Model file for the job. Use its own axes, mm. A direction names the side the tool comes from. Round coordinates to 2 decimals unless told otherwise and drop trailing zeros. Loops run counter-clockwise (first coordinate to the right, second up) from the corner with the lowest first, then second, coordinate; pieces in that order, holes last. Notation, with made-up numbers: (54, 22.5) - (107, 22.5) arc R17 cw to (107, 27.5) - close; hole circle Ø11 at (32.25, -37). An arc over 180 degrees is marked (long way). Answer as a JSON object with one key per item and string values.
from build123d import *

# Parameters (mm, degrees)
F3_DEPTH  = 533.4
F5_DEPTH  = 330.2
F6_W      = 895.4597115517
F6_H      = 69.037437439
F7_DEPTH  = 254
F9_DEPTH  = 152.4
F11_W     = 951.6055583954
F11_H     = 58.4162473679
F12_DEPTH = 254
F13_R     = 205.1226496696
F14_DEPTH = 203.2
F16_DEPTH = 203.2
F17_W     = 673.4294295311
F17_H     = 270.8390951157
F18_DEPTH = 254
F20_DEPTH = 228.6
F22_DEPTH = 50.8
F23_W     = 39.8923233151
F23_H     = 31.9777131081
F24_DEPTH = 50.8
F25_R     = 128.4316644383
F26_DEPTH = 25.4


with BuildPart() as f3:
    # F2 (on face) → F3 (new body, symmetric)
    with BuildSketch(Plane.YZ):
        Polygon((580.4695487022, 438.6440515518), (954.6338915825, 438.6440515518), (954.6338915825, 557.7040910721), (517.2948241234, 520.7), (458.9797258377, 382.7587366104), (145.5359309912, 382.7587366104), (-36.6988368332, 411.9162857533), (-36.6988368332, 297.7158427238), (553.741812706, 297.7158427238), align=None)
    extrude(amount=F3_DEPTH, both=True)

    # F4 (on face) → F5 (join, symmetric)
    with BuildSketch(Plane.YZ):
        Polygon((145.5359309912, 382.7587366104), (228.7405356924, 382.7587366104), (262.6523375511, 594.7075978799), (262.6523375511, 840.8291935921), (154.4104069471, 914.7086143494), (-513.9405727386, 864.883005619), (-623.9005923271, 818.4935450554), (-678.880572319, 583.110332489), (-653.1087756157, 419.8883771896), (-603.2831072807, 382.7587366104), align=None)
    extrude(amount=F5_DEPTH, both=True)

    # F6 (on face) → F7 (join)
    with BuildSketch(Plane(origin=(0, 0, 382.7587366104), x_dir=(1, 0, 0), z_dir=(0, 0, -1))):
        with Locations((0, 352.2024452686)):
            Rectangle(F6_W, F6_H)
    extrude(amount=F7_DEPTH)

    # F8 (on face) → F9 (join)
    with BuildSketch(Plane(origin=(-447.7298557758, 0, 0), x_dir=(0, -1, 0), z_dir=(-1, 0, 0))):
        with BuildLine():
            ThreePointArc((350.7186164637, 0), (482.3983530717, 54.5435321866), (536.9418859482, 186.2232685089))
            ThreePointArc((536.9418859482, 186.2232685089), (219.0388818068, 317.9030048312), (350.7186164637, 0))
        make_face()
    extrude(amount=F9_DEPTH)

    # F10: F3 across face


with BuildPart() as f3_1:
    add(f3.part)
    add(f3.part.mirror(Plane.YZ))

    # F11 (on face) → F12 (join)
    with BuildSketch(Plane(origin=(0, 0, 438.6440515518), x_dir=(1, 0, 0), z_dir=(0, 0, -1))):
        with Locations((0, -776.2938737869)):
            Rectangle(F11_W, F11_H)
    extrude(amount=F12_DEPTH)

    # F13 (on face) → F14 (join)
    with BuildSketch(Plane(origin=(-475.8027791977, 0, 0), x_dir=(0, -1, 0), z_dir=(-1, 0, 0))):
        with Locations((-747.085750103, 205.1226496696)):
            Circle(F13_R)
    extrude(amount=F14_DEPTH)

    # F15 (on face) → F16 (join)
    with BuildSketch(Plane.YZ.offset(475.8027791977)):
        with BuildLine():
            ThreePointArc((747.085750103, 410.2452993393), (602.0421335466, 60.0790331133), (952.2083997726, 205.1226496696))
            ThreePointArc((952.2083997726, 205.1226496696), (911.4904289466, 327.7864299058), (805.5019974709, 401.751344043))
            ThreePointArc((805.5019974709, 401.751344043), (776.6010225612, 408.1107037497), (747.085750103, 410.2452993393))
        make_face()
    extrude(amount=F16_DEPTH)

    # F17 (on face) → F18 (join)
    with BuildSketch(Plane(origin=(0, 0, 438.6440515518), x_dir=(1, 0, 0), z_dir=(0, 0, -1))):
        with Locations((0, -784.2597365379)):
            Rectangle(F17_W, F17_H)
    extrude(amount=-F18_DEPTH)

    # F19 (on face) → F20 (join, symmetric)
    with BuildSketch(Plane.YZ):
        Polygon((630.3312778473, 775.7710305214), (648.8401889801, 692.6440515518), (919.6792840958, 692.6440515518), (939.593911171, 959.6104708672), (900.0770449638, 978.5098520279), (850.2513766289, 758.5897532463), align=None)
    extrude(amount=F20_DEPTH, both=True)

    # F21 (on face) → F22 (join, symmetric)
    with BuildSketch(Plane.YZ):
        Polygon((224.0662593073, 867.1657259695), (262.6523375511, 840.8291935921), (262.6523375511, 813.3391737938), (304.5946338236, 901.0808301074), (265.4504130698, 927.7983169367), align=None)
    extrude(amount=F22_DEPTH, both=True)

    # F23 (on face) → F24 (join)
    with BuildSketch(Plane(origin=(0, 516.3670714777, 756.5377224693), x_dir=(1, 0, 0), z_dir=(0, 0.5637436051, 0.8259498458))):
        with Locations((0, -278.8930535316)):
            Rectangle(F23_W, F23_H)
    extrude(amount=F24_DEPTH)

    # F25 (on face) → F26 (join)
    with BuildSketch(Plane(origin=(0, 545.005246616, 798.4959746344), x_dir=(1, 0, 0), z_dir=(0, 0.5637436051, 0.8259498458))):
        with Locations((0, -278.8930535316)):
            Circle(F25_R)
    extrude(amount=F26_DEPTH)


solid = f3_1.part
1) Two-plate mould, pull along Y, no slides. Class faces 1 (the flat face through (4.623, -175.087, 890.145)), 2 (the flat face through (-430.378, 55.694, 397.133)), 3 (the flat face through (679.003, 744, 208)): pulls with the +Y half, pulls with the -Y half, needs draft (parallel to the pull), parting line crosses it, or undercut.
Values follow:
{"face 1": "pulls with the -Y half", "face 2": "undercut", "face 3": "needs draft"}
2) Probe probe 1 along X at (y, z) = (752, 84.5); probe 2 along Y at (x, z) = (-526.5, 331.5); probe 3 along Z at (x, y) = (73, -484.5). List the from-to ranges inside material, lowest first.
Values follow:
{"probe 1": "-679 to -475.8, 475.8 to 679", "probe 2": "-467.23 to -234.21, -36.7 to 560.15, 585.52 to 908.65", "probe 3": "382.76 to 867.08"}
3) Drop flat-ended pins along their axis: P1, Ø3, axis at x = -478, z = 401, coming from the -Y side; P2, Ø12, axis at x = 454.5, y = -302.5, coming from the +Z side; P3, Ø3, axis at y = 576, z = 431.5, coming from the -X side. Give the stop position or say it passes through.
Values follow:
{"P1": "y = -36.7", "P2": "z = 367.6", "P3": "x = -533.4"}
4) Tool access for faces 4 (the flat face through (3.2, 639.456, 734.789)), 5 (the flat face through (228.6, 817, 742)), 6 (the flat face through (0.711, 272.248, 923.158)): list every direction of +Z, -Z, +X, -X, +Y, -Y with a clear straight run to the whole face (end or side of a thin tool).
Values follow:
{"face 4": "+X, -X", "face 5": "+Z, +X, +Y", "face 6": "none"}
5) Slice it at D-D on y = 15. List the corners of the cut face in (x, z).
Values follow:
{"outline": "(-533.4, 297.72) - (533.4, 297.72) - (533.4, 403.64) - (330.2, 403.64) - (330.2, 904.32) - (-330.2, 904.32) - (-330.2, 403.64) - (-533.4, 403.64) - close"}
6) Slice it at A-A on x = -407. List the corners of the cut face in (y, z).
Values follow:
{"outline": "(-386.72, 128.76) - (-317.68, 128.76) - (-317.68, 382.76) - (-386.72, 382.76) - close; (-36.7, 297.72) - (553.74, 297.72) - (580.47, 438.64) - (747.09, 438.64) - (747.09, 184.64) - (805.5, 184.64) - (805.5, 438.64) - (954.63, 438.64) - (954.63, 557.7) - (517.29, 520.7) - (458.98, 382.76) - (145.54, 382.76) - (-36.7, 411.92) - close"}
7) Slice it at B-B on z = 661. List the corners of the cut face in (x, y), then the cut area to 3 significant figures.
Values follow:
{"outline": "(-336.71, 648.84) - (336.71, 648.84) - (336.71, 919.68) - (-336.71, 919.68) - close; (-330.2, -660.69) - (330.2, -660.69) - (330.2, 262.65) - (-330.2, 262.65) - close", "area": "792,000 mm²"}
